Read the model definition and answer for the solid it produces. Units are mm, in the model's axes. A direction names the side the tool comes from. Coordinates: 2 decimals unless noted, no trailing zeros. Order: outer loops, then holes, each group sorted by start corner. A loop starts at its lowest first (then second) coordinate and runs counter-clockwise, first axis right, second up. Notation, with made-up numbers: (35, -25) -> (39, -25) arc R15 ccw to (39, -11) -> close; hole circle Ø3 at (-14.5, 34.5). An arc over 180 degrees is marked (long way). Answer in a Markdown table with one row per item.
from build123d import *

# Parameters (mm, degrees)
SKETCH1_W                                            = 25
SKETCH1_H                                            = 37
BOSS_EXTRUDE2_DEPTH                                  = 20
SKETCH4_W                                            = 23.2
SKETCH4_H                                            = 35.3
CUT_EXTRUDE1_DEPTH                                   = 18
SKETCH30_W                                           = 10
SKETCH30_H                                           = 10
BOSS_EXTRUDE5_DEPTH                                  = 3
CBORE_FOR_M3_HEXAGON_HEAD_BOLTS_FULL_THR_D           = 3.4
CBORE_FOR_M3_HEXAGON_HEAD_BOLTS_FULL_THR_CBORE_D     = 9
CBORE_FOR_M3_HEXAGON_HEAD_BOLTS_FULL_THR_CBORE_DEPTH = 0.5


with BuildPart() as part:
    # Sketch1 → Boss-Extrude2 (new body)
    with BuildSketch(Plane(origin=(0, 0, 0), x_dir=(1, 0, 0), z_dir=(0, 1, 0))):
        with Locations((-76.226170177, 10.94482429)):
            Rectangle(SKETCH1_W, SKETCH1_H)
    extrude(amount=BOSS_EXTRUDE2_DEPTH)

    # Sketch4 → Cut-Extrude1 (cut)
    with BuildSketch(Plane(origin=(0, 20, 0), x_dir=(1, 0, 0), z_dir=(0, 1, 0))):
        with Locations((-76.226170177, 10.94482429)):
            Rectangle(SKETCH4_W, SKETCH4_H)
    extrude(amount=-CUT_EXTRUDE1_DEPTH, mode=Mode.SUBTRACT)

    # Sketch30 → Boss-Extrude5 (add)
    with BuildSketch(Plane.ZY.offset(88.726170177)):
        with Locations((-34.44482429, 10)):
            Rectangle(SKETCH30_W, SKETCH30_H)
        with Locations((12.55517571, 10)):
            Rectangle(SKETCH30_W, SKETCH30_H)
    extrude(amount=-BOSS_EXTRUDE5_DEPTH)

    # CBORE for M3 Hexagon head bolts-Full thread-grades AB5 (through all)
    with Locations(Plane(origin=(-85.726170177, 10, -34.44482429), x_dir=(0, 0, 1), z_dir=(1, 0, 0))):
        with Locations((0, 0), (47, 0)):
            CounterBoreHole(CBORE_FOR_M3_HEXAGON_HEAD_BOLTS_FULL_THR_D / 2, CBORE_FOR_M3_HEXAGON_HEAD_BOLTS_FULL_THR_CBORE_D / 2, CBORE_FOR_M3_HEXAGON_HEAD_BOLTS_FULL_THR_CBORE_DEPTH)


solid = part.part
Q1. The part is cut by section B-B (y = 18.25). Write down the section's boundary in (x, z).
Outcome:
| item | result |
|---|---|
| outline | (-88.73, -29.44) -> (-63.73, -29.44) -> (-63.73, 7.56) -> (-88.73, 7.56) -> close; hole (-87.83, -28.59) -> (-64.63, -28.59) -> (-64.63, 6.71) -> (-87.83, 6.71) -> close |
Q2. The part is cut by section A-A (y = 10). Write down the section's boundary in (x, z).
Outcome:
| item | result |
|---|---|
| outline | (-88.73, -39.44) -> (-85.73, -39.44) -> (-85.73, -38.94) -> (-86.23, -38.94) -> (-86.23, -36.14) -> (-88.73, -36.14) -> close; (-88.73, -32.74) -> (-86.23, -32.74) -> (-86.23, -29.94) -> (-85.73, -29.94) -> (-85.73, -29.44) -> (-63.73, -29.44) -> (-63.73, 7.56) -> (-85.73, 7.56) -> (-85.73, 8.06) -> (-86.23, 8.06) -> (-86.23, 10.86) -> (-88.73, 10.86) -> close; (-88.73, 14.26) -> (-86.23, 14.26) -> (-86.23, 17.06) -> (-85.73, 17.06) -> (-85.73, 17.56) -> (-88.73, 17.56) -> close; hole (-87.83, -28.59) -> (-64.63, -28.59) -> (-64.63, 6.71) -> (-87.83, 6.71) -> close |
Q3. The part is cut by section C-C (x = -68.75). Write down the section's boundary in (y, z).
Outcome:
| item | result |
|---|---|
| outline | (0, -29.44) -> (20, -29.44) -> (20, -28.59) -> (2, -28.59) -> (2, 6.71) -> (20, 6.71) -> (20, 7.56) -> (0, 7.56) -> close |
Q4. Given pin 1 (2.5 mm diameter, centred on x = -87, z = 14, fed in from +Y); pin 2 (4 mm diameter, centred on y = 10, z = -34.44, fed in from +X); pin 3 (9 mm diameter, centred on x = -77, y = 9.5, fed in from +Z), each flat-ended and moving along its own axis, determine where each tip first touches the part or whether it passes through.
Outcome:
| item | result |
|---|---|
| pin 1 | y = 15 |
| pin 2 | x = -86.23 |
| pin 3 | z = 7.56 |
Q5. For a pull along X with two mould halves and no side action, classify faces 1 (the face through (-76, 11, -28.595)), 2 (the face through (-76, 11, 6.705)), 3 (the face through (-85.726, 11, -39)), 4 (the face through (-76, 10, -29.445)) as pulls with the +X half, pulls with the -X half, needs draft (parallel to the pull), parting line crosses it, or undercut.
Outcome:
| item | result |
|---|---|
| face 1 | undercut |
| face 2 | undercut |
| face 3 | pulls with the +X half |
| face 4 | needs draft |
Q6. For faces 5 (the face through (-87.826, 11, -11)), 6 (the face through (-85.726, 11, 8)), 7 (the face through (-87, 15, -35)), 8 (the face through (-86.226, 12, 12)), 9 (the face through (-87, 5, 12)), determine the directions among +Z, -Z, +X, -X, +Y, -Y from which every point of the face is accessible in a straight line to the end or side of a thin tool.
Outcome:
| item | result |
|---|---|
| face 5 | +Y |
| face 6 | +Z, +X, +Y, -Y |
| face 7 | -Z, +X, -X, +Y |
| face 8 | +X |
| face 9 | +Z, +X, -X, -Y |
Q7. The part is cut by section D-D (z = -6). Write down the section's boundary in (x, y).
Outcome:
| item | result |
|---|---|
| outline | (-88.73, 0) -> (-63.73, 0) -> (-63.73, 20) -> (-64.63, 20) -> (-64.63, 2) -> (-87.83, 2) -> (-87.83, 20) -> (-88.73, 20) -> close |
Q8. Consider line 1 (Z direction, x = -87.15, y = 10); line 2 (Z direction, x = -70, y = 4.5); line 3 (X direction, y = 16.5, z = -13). Determine where each line is inside the solid, lowest interval first.
Outcome:
| item | result |
|---|---|
| line 1 | -39.44 to -36.14, -32.74 to -28.59, 6.71 to 10.86, 14.26 to 17.56 |
| line 2 | -29.44 to -28.59, 6.71 to 7.56 |
| line 3 | -88.73 to -87.83, -64.63 to -63.73 |
